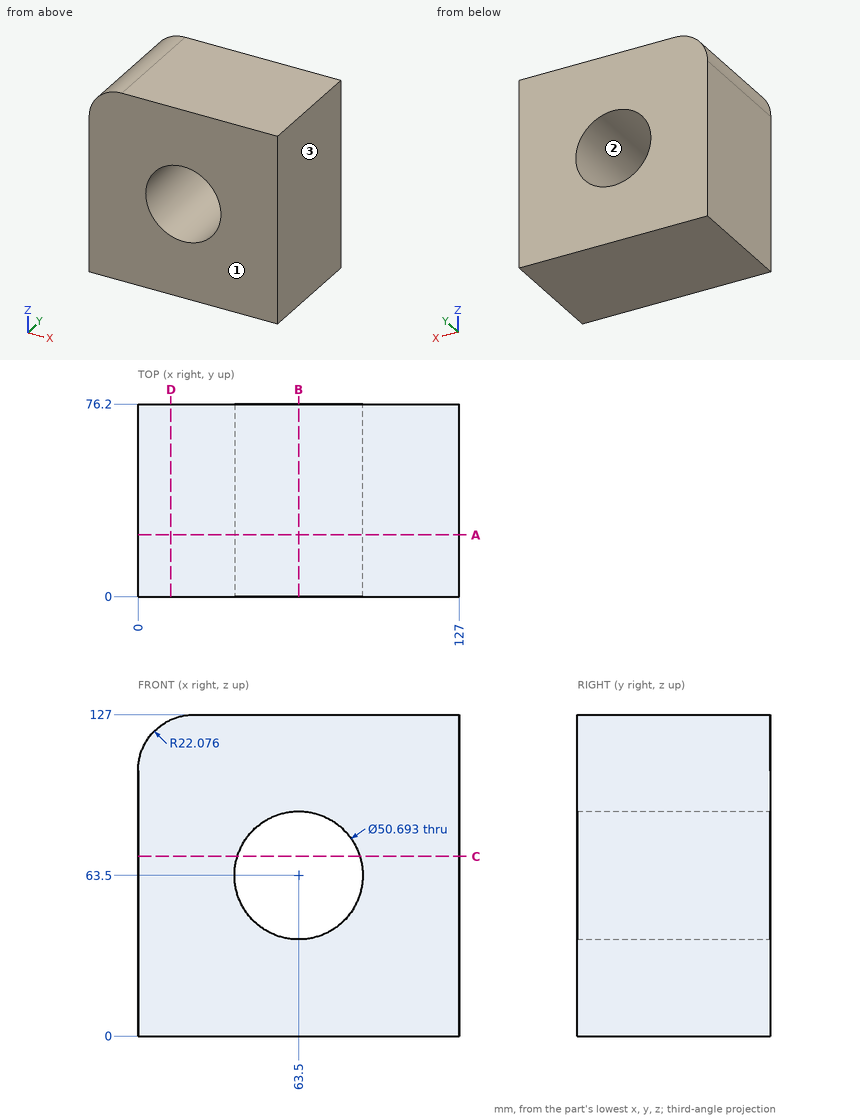
Verification items for this drawing (mm, ordinates from the low corner). Coordinates: 2 decimals unless noted, no trailing zeros. Write each loop counter-clockwise with the first axis right and the second up, starting at its lowest first coordinate (ties: lowest second). Pieces come first, ordered by that corner, then holes. Notation, with made-up numbers: M 89.25,58 L 102.25,58 A19 ccw 102.25,68 Z; hole C 22.5,-10.75 d10. An arc over 180 degrees is marked long. Answer as a JSON object with one key per item and string values. Group by question number.
(1) Material ranges on line 1 (Z direction, x = 63.5, y = 31.5); line 2 (X direction, y = 73, z = 74); line 3 (X direction, y = 52.5, z = 45.5) (1 decimal), recorded low to high.
(2) Cross-section at B-B, the plane x = 63.5. Record the cut outline in (y, z).
(3) Cross-section at A-A, the plane y = 24.5. Record the cut outline in (x, z) (1 decimal).
(4) Gauge pin test, flat end, axial feed: pin 1 (10 mm diameter, centred on x = 79.5, z = 75.5, fed in from -Y). Record the tip position at first contact, or that the pin passes through.
(5) Cross-section at C-C, the plane z = 71. Record the cut outline in (x, y), and give its area (3 significant figures).
(6) Release check for a two-part mould opening along X. For the marked faces 1, 2 and 3 record: +X half, -X half, draft (parallel to the pull), parting line (faces both ways), or undercut.
(7) Cross-section at D-D, the plane x = 13. Record the cut outline in (y, z).
Reply:
{
 "1": {"line 1": "0 to 38.15, 88.85 to 127", "line 2": "0 to 40.43, 86.57 to 127", "line 3": "0 to 45.7, 81.3 to 127"},
 "2": {"outline": "M 0,0 L 76.2,0 L 76.2,38.15 L 0,38.15 Z; M 0,88.85 L 76.2,88.85 L 76.2,127 L 0,127 Z"},
 "3": {"outline": "M 0,0 L 127,0 L 127,127 L 22.1,127 A22.1 ccw 0,104.9 Z; hole C 63.5,63.5 d50.7"},
 "4": {"pin 1": "through"},
 "5": {"outline": "M 0,0 L 39.29,0 L 39.29,76.2 L 0,76.2 Z; M 87.71,0 L 127,0 L 127,76.2 L 87.71,76.2 Z", "area": "5,990 mm²"},
 "6": {"face 1": "draft", "face 2": "undercut", "face 3": "+X half"},
 "7": {"outline": "M 0,0 L 76.2,0 L 76.2,125.05 L 0,125.05 Z"}
}
